from build123d import *

# Parameters (mm, degrees)
SKETCH_W        = 120
SKETCH_H        = 290
PAD_DEPTH       = 140
SKETCH001_W     = 120
SKETCH001_H     = 170
POCKET_DEPTH    = 100
POCKET001_DEPTH = 120.001
SKETCH003_R     = 15
POCKET002_DEPTH = 120.001
POCKET003_DEPTH = 290.001
SKETCH005_W     = 120
SKETCH005_H     = 30
POCKET004_DEPTH = 20
POCKET005_DEPTH = 40.001
POCKET006_DEPTH = 10


with BuildPart() as part:
    # Sketch → Pad (new body)
    with BuildSketch(Plane.XY):
        Rectangle(SKETCH_W, SKETCH_H)
    extrude(amount=PAD_DEPTH)

    # Sketch001 → Pocket (cut)
    with BuildSketch(Plane.XY.offset(140)):
        with Locations((0, -60)):
            Rectangle(SKETCH001_W, SKETCH001_H)
    extrude(amount=-POCKET_DEPTH, mode=Mode.SUBTRACT)

    # Sketch002 → Pocket001 (cut, through all)
    with BuildSketch(Plane.XZ.offset(-25)):
        Polygon((40, 140), (60, 65), (60, 140), align=None)
        Polygon((-60, 65), (-40, 140), (-60, 140), align=None)
    extrude(amount=-POCKET001_DEPTH, mode=Mode.SUBTRACT)

    # Sketch003 → Pocket002 (cut, through all)
    with BuildSketch(Plane.XZ.offset(-25)):
        with Locations((-26, 65)):
            Circle(SKETCH003_R)
        with Locations((26, 65)):
            Circle(SKETCH003_R)
        with BuildLine():
            ThreePointArc((-22.499959, 125), (-37.5, 110.000021), (-22.5, 95))
            Line((-22.5, 95), (22.5, 95))
            ThreePointArc((22.5, 95), (37.5, 110.000021), (22.499959, 125))
            Line((-22.499959, 125), (22.499959, 125))
        make_face()
    extrude(amount=-POCKET002_DEPTH, mode=Mode.SUBTRACT)

    # Sketch004 → Pocket003 (cut, through all)
    with BuildSketch(Plane.XZ.offset(145)):
        Polygon((-60, 30), (-46.01077, 0), (-60, 0), align=None)
        Polygon((60, 30), (46.01077, 0), (60, 0), align=None)
    extrude(amount=-POCKET003_DEPTH, mode=Mode.SUBTRACT)

    # Sketch005 → Pocket004 (cut)
    with BuildSketch(Plane(origin=(0, 145, 0), x_dir=(-1, 0, 0), z_dir=(0, 1, 0))):
        with Locations((0, 15)):
            Rectangle(SKETCH005_W, SKETCH005_H)
    extrude(amount=-POCKET004_DEPTH, mode=Mode.SUBTRACT)

    # Sketch006 → Pocket005 (cut, through all)
    with BuildSketch(Plane.XY.offset(40)):
        with BuildLine():
            ThreePointArc((15, -24.999997), (-2.5e-05, -10), (-15, -25.000048))
            Line((-15, -80.000045), (-15, -25.000048))
            ThreePointArc((-15, -80.000045), (2.3e-05, -95), (15, -79.999998))
            Line((15, -24.999997), (15, -79.999998))
        make_face()
    extrude(amount=-POCKET005_DEPTH, mode=Mode.SUBTRACT)

    # Sketch007 → Pocket006 (cut)
    with BuildSketch(Plane.XY.offset(40)):
        with BuildLine():
            ThreePointArc((35, -25), (-2.1e-05, 10), (-35, -25.000043))
            Line((-35, -25.000043), (-35, -79.999957))
            ThreePointArc((-35, -79.999957), (-2.1e-05, -115), (35, -80))
            Line((35, -25), (35, -80))
        make_face()
    extrude(amount=-POCKET006_DEPTH, mode=Mode.SUBTRACT)


solid = part.part
Input: part model. Units: mm. Frame: model coordinates. A direction names the side the tool comes from. Give positions to 0.01 mm unless a question says otherwise; leave off trailing zeros. Loops run counter-clockwise (first coordinate to the right, second up) from the corner with the lowest first, then second, coordinate; pieces in that order, holes last. Notation, with made-up numbers: M 41,42.25 L 67,42.25 A16 cw 67,71.25 Z; hole C 56,55.5 d9. An arc over 180 degrees is marked long. Use CSV: the item, a comma, the result in double quotes.
(1) Pin query (flat end, axial travel): P1, Ø10, axis at x = -36.5, z = 118.5, coming from the -Y side; P2, Ø2, axis at y = 96.5, z = 68, coming from the -X side; P3, Ø24, axis at y = -58.5, z = 15.5, coming from the +X side. Return the tip coordinate at first contact, or that it passes through.
Outcome:
P1,"stops at y = 25"
P2,"stops at x = -59.47"
P3,"stops at x = 58.83"
(2) Material intervals for L1, parallel to Z at x = -26, y = 113.5; L2, parallel to X at y = -48.5, z = 39.5; L3, parallel to Z at x = -2.5, y = 89, sorted ascending. Write a range as [from, to].
Outcome:
L1,"z = [0, 50], [80, 95.41], [124.59, 140]"
L2,"x = [-60, -35], [35, 60]"
L3,"z = [0, 95], [125, 140]"
(3) Section A-A, the plane y = -39.5. Return loops of the section in (x, z), plus the area to 3 significant figures.
Outcome:
outline,"M -60,30 L -46.01,0 L -15,0 L -15,30 L -35,30 L -35,40 L -60,40 Z; M 15,0 L 46.01,0 L 60,30 L 60,40 L 35,40 L 35,30 L 15,30 Z"
area,"2,780 mm²"
(4) Section C-C, the plane z = 110. Return loops of the section in (x, y).
Outcome:
outline,"M -48,25 L -37.5,25 L -37.5,145 L -48,145 Z; M 37.5,25 L 48,25 L 48,145 L 37.5,145 Z"
(5) Pull-direction query (Y, two-part tool) for faces 6 (the face through (-35, -52, 35)), 7 (the face through (37.496, 84.16, 109.67)), 8 (the face through (-1, -145, 20)); classes: pulls with the +Y half, pulls with the -Y half, needs draft (parallel to the pull), parting line crosses it, or undercut.
Outcome:
face 6,"undercut"
face 7,"needs draft"
face 8,"pulls with the -Y half"
(6) Set-up query: faces 1 (the face through (1, 135, 30)), 2 (the face through (60, 30, 43)), 3 (the face through (0.77, 9.99, 35.07)), 4 (the face through (-41, -59, 40)), 5 (the face through (0, 84, 125)). Return all of +Z, -Z, +X, -X, +Y, -Y with unobstructed straight access to the full face (end or side cutting, diameter ignored); none if empty.
Outcome:
face 1,"-Z, +X, -X, +Y"
face 2,"+Z, -Z, +X, +Y, -Y"
face 3,"+Z"
face 4,"+Z, +X, -X, -Y"
face 5,"+Y, -Y"
(7) Section D-D, the plane y = 90. Return loops of the section in (x, z).
Outcome:
outline,"M -60,30 L -46.01,0 L 46.01,0 L 60,30 L 60,65 L 40,140 L -40,140 L -60,65 Z; hole C -26,65 d30; hole M -22.5,95 L 22.5,95 A15 ccw 22.5,125 L -22.5,125 A15 ccw Z; hole C 26,65 d30"
(8) Section B-B, the plane x = 0. Return loops of the section in (y, z).
Outcome:
outline,"M -145,0 L -95,0 L -95,30 L -115,30 L -115,40 L -145,40 Z; M -10,0 L 125,0 L 125,30 L 145,30 L 145,95 L 25,95 L 25,40 L 10,40 L 10,30 L -10,30 Z; M 25,125 L 145,125 L 145,140 L 25,140 Z"
